Check sheet for the modelled part. Datum: model origin and axes. Units: mm. Face numbers are marked on the shaded views. A direction names the side the tool comes from. Give positions to 0.01 mm unless a question says otherwise; leave off trailing zeros. Order: outer loops, then holes, each group sorted by start corner. A loop starts at its lowest first (then second) coordinate and runs counter-clockwise, first axis right, second up. Notation, with made-up numbers: (40, 73.5) -> (65, 73.5) arc R26 ccw to (65, 105.5) -> close; hole circle Ø9 at (87.25, -31). An arc over 180 degrees is marked (long way). Answer in a Markdown table with one row per item. Add a question column.
(1) Set-up check for the marked faces 4, 5 and 6: record each of +Z, -Z, +X, -X, +Y, -Y from which the full face is reachable in a straight line by a thin tool's end or side.
(2) Cross-section at C-C (z = -20). Record the cut outline in (x, y).
(3) Thickness scan on L1, parallel to X at y = 5.75, z = 20; L2, parallel to X at y = 9, z = -36; L3, parallel to Y at x = 50.5, z = -40. Record the ranges inside material, lowest first. Write a range as [from, to].
(4) Release check for a two-part mould opening along X. For the marked faces 1, 2 and 3 record: released by +X, released by -X, zero draft, split by the parting line, or undercut.
(5) Cross-section at B-B (x = 32.5). Record the cut outline in (y, z).
(6) Cross-section at A-A (z = 20). Record the cut outline in (x, y).
(7) Go/stop test with flat-tipped pins: pin 1 (3.5 mm diameter, centred on x = 50.5, y = 1.5, fed in from -Z); pin 2 (5 mm diameter, centred on x = -25.5, z = -34.5, fed in from -Y); pin 3 (11 mm diameter, centred on x = -42.5, y = 19.5, fed in from +Z); pin 4 (1.5 mm diameter, centred on x = -30, z = -8.5, fed in from -Y). Record where each tip stops, or that it passes through.
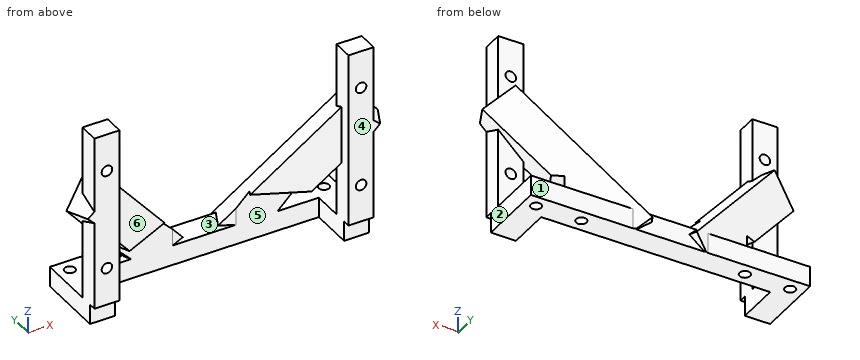
```python
from build123d import *

# Parameters (mm, degrees)
SKETCH_1_W          = 10
SKETCH_1_H          = 70
SKETCH_1_R          = 2.1
EXTRUDE_1_DEPTH     = 8
EXTRUDE_1_2_DEPTH   = 8
SKETCH_2_W          = 10
SKETCH_2_H          = 8
EXTRUDE_2_DEPTH     = 30
SKETCH_4_W          = 8
SKETCH_4_H          = 10
EXTRUDE_3_DEPTH     = 97
SKETCH_6_R          = 2.1
CUT_EXTRUDE_1_DEPTH = 101.320735643
EXTRUDE_4_DEPTH     = 10
SKETCH_11_W         = 111
SKETCH_11_H         = 6
CUT_EXTRUDE_3_DEPTH = 86.153989901
CUT_EXTRUDE_5_DEPTH = 20
SKETCH_13_W         = 8
SKETCH_13_H         = 3
CUT_EXTRUDE_7_DEPTH = 130.217721636
SKETCH_14_W         = 130
SKETCH_14_H         = 5
CUT_EXTRUDE_8_DEPTH = 105.816357447


with BuildPart() as part:
    # Sketch 1 → Extrude 1 (new body)
    with BuildSketch(Plane(origin=(0, 0, 0), x_dir=(1, 0, 0), z_dir=(0, 1, 0))):
        with Locations((-50.5, 0)):
            Rectangle(SKETCH_1_W, SKETCH_1_H)
        with Locations(Location((-50.5, 20, 0), (0, 0, 270))):
            Circle(SKETCH_1_R, mode=Mode.SUBTRACT)
        with Locations(Location((-50.5, -20, 0), (0, 0, 90))):
            Circle(SKETCH_1_R, mode=Mode.SUBTRACT)
    extrude(amount=EXTRUDE_1_DEPTH)



with BuildPart() as body_2:
    # Sketch 1 → Extrude 1 2 (new body)
    with BuildSketch(Plane(origin=(0, 0, 0), x_dir=(1, 0, 0), z_dir=(0, 1, 0))):
        with Locations((50.5, 0)):
            Rectangle(SKETCH_1_W, SKETCH_1_H)
        with Locations(Location((50.5, -20, 0), (0, 0, 270))):
            Circle(SKETCH_1_R, mode=Mode.SUBTRACT)
        with Locations(Location((50.5, 20, 0), (0, 0, 90))):
            Circle(SKETCH_1_R, mode=Mode.SUBTRACT)
    extrude(amount=EXTRUDE_1_2_DEPTH)


with BuildPart() as part_1:
    add(part.part)

    add(body_2.part)  # Extrude 2 merges body 2
    # Sketch 2 → Extrude 2 (add)
    with BuildSketch(Plane(origin=(0, 0, 0), x_dir=(1, 0, 0), z_dir=(0, 1, 0))):
        with Locations((-50.5, 39)):
            Rectangle(SKETCH_2_W, SKETCH_2_H)
        with Locations((50.5, 39)):
            Rectangle(SKETCH_2_W, SKETCH_2_H)
    extrude(amount=EXTRUDE_2_DEPTH)

    # Sketch 4 → Extrude 3 (add)
    with BuildSketch(Plane.ZY.offset(-45.5)):
        with Locations((-39, 25)):
            Rectangle(SKETCH_4_W, SKETCH_4_H)
    extrude(amount=EXTRUDE_3_DEPTH)

    # Sketch 6 → Cut-Extrude 1 (cut, through all)
    with BuildSketch(Plane(origin=(0, 0, -43), x_dir=(-1, 0, 0), z_dir=(0, 0, -1))):
        with Locations((-50.5, 25)):
            Circle(SKETCH_6_R)
        with Locations((-32.5, 25)):
            Circle(SKETCH_6_R)
        with Locations((32.5, 25)):
            Circle(SKETCH_6_R)
        with Locations((50.5, 25)):
            Circle(SKETCH_6_R)
    extrude(amount=-CUT_EXTRUDE_1_DEPTH, mode=Mode.SUBTRACT)

    # Sketch 9 → Extrude 4 (add)
    with BuildSketch(Plane(origin=(-9.912643831, 21.257733297, 0), x_dir=(0, 0, 1), z_dir=(-0.4226182617407003, 0.9063077870366496, 0))):
        Polygon((13.243149515, -41.193317821), (-37.922770357, 5.903700872), (-48.463730846, -5.547935659), (2.702189027, -52.644954352), align=None)
    extrude_4 = extrude(amount=EXTRUDE_4_DEPTH)

    # Mirror 2: Extrude 4 across plane
    add(extrude_4.mirror(Plane(origin=(0, 0, 0), x_dir=(0, 0, 1), z_dir=(1, 0, 0))))

    # Sketch 11 → Cut-Extrude 3 (cut, through all)
    with BuildSketch(Plane(origin=(0, 0, 0), x_dir=(1, 0, 0), z_dir=(0, 1, 0))):
        with Locations((0, 46)):
            Rectangle(SKETCH_11_W, SKETCH_11_H)
    extrude(amount=CUT_EXTRUDE_3_DEPTH, mode=Mode.SUBTRACT)

    # Sketch 12 → Cut-Extrude 5 (cut)
    with BuildSketch(Plane(origin=(0, 0, -43), x_dir=(-1, 0, 0), z_dir=(0, 0, -1))):
        Polygon((-45.5, 20), (-45.5, 0), (-60, 0), (-60, -5), (60, -5), (60, 0), (45.5, 0), (45.5, 20), align=None)
    extrude(amount=-CUT_EXTRUDE_5_DEPTH, mode=Mode.SUBTRACT)

    # Sketch 13 → Cut-Extrude 7 (cut, through all)
    with BuildSketch(Plane.ZY.offset(55.5)):
        with Locations((-39, 1.5)):
            Rectangle(SKETCH_13_W, SKETCH_13_H)
    extrude(amount=-CUT_EXTRUDE_7_DEPTH, mode=Mode.SUBTRACT)

    # Sketch 14 → Cut-Extrude 8 (cut, through all)
    with BuildSketch(Plane(origin=(0, 0, -43), x_dir=(-1, 0, 0), z_dir=(0, 0, -1))):
        with Locations((0, -2.5)):
            Rectangle(SKETCH_14_W, SKETCH_14_H)
    extrude(amount=-CUT_EXTRUDE_8_DEPTH, mode=Mode.SUBTRACT)


solid = part_1.part
```
Answer below:
| question | item | result |
|---|---|---|
| 1 | face 4 | +Z, -Z, +X, -X, -Y |
| 1 | face 5 | -Z, -Y |
| 1 | face 6 | +Z, -Z, -Y |
| 2 | outline | (-55.5, 0) -> (-52.6, 0) -> (-52.6, 8) -> (-55.5, 8) -> close; (-48.4, 0) -> (-45.5, 0) -> (-45.5, 8) -> (-48.4, 8) -> close; (-42.91, 16.9) -> (-38.69, 7.84) -> (-19.51, 16.78) -> (-23.74, 25.84) -> close; (19.51, 16.78) -> (38.69, 7.84) -> (42.91, 16.9) -> (23.74, 25.84) -> close; (45.5, 0) -> (48.4, 0) -> (48.4, 8) -> (45.5, 8) -> close; (52.6, 0) -> (55.5, 0) -> (55.5, 8) -> (52.6, 8) -> close |
| 3 | L1 | x = [-55.5, -52.6], [-48.4, -45.5], [45.5, 48.4], [52.6, 55.5] |
| 3 | L2 | x = [-55.5, -45.5], [45.5, 55.5] |
| 3 | L3 | y = [3, 22.9], [27.1, 30] |
| 4 | face 1 | zero draft |
| 4 | face 2 | released by +X |
| 4 | face 3 | undercut |
| 5 | outline | (10.73, -23) -> (20, -23) -> (20, -31.67) -> (21.76, -32.48) -> (21.76, -9.5) -> (10.73, -4.43) -> close; (20, -43) -> (22.9, -43) -> (22.9, -35) -> (20, -35) -> close; (27.1, -43) -> (30, -43) -> (30, -35) -> (27.1, -35) -> close |
| 6 | outline | (-55.5, 0) -> (-52.6, 0) -> (-52.6, 8) -> (-55.5, 8) -> close; (-48.4, 0) -> (-45.5, 0) -> (-45.5, 8) -> (-48.4, 8) -> close; (45.5, 0) -> (48.4, 0) -> (48.4, 8) -> (45.5, 8) -> close; (52.6, 0) -> (55.5, 0) -> (55.5, 8) -> (52.6, 8) -> close |
| 7 | pin 1 | stops at z = -43 |
| 7 | pin 2 | stops at y = 20 |
| 7 | pin 3 | stops at z = 6.87 |
| 7 | pin 4 | stops at y = 11.54 |
